```python
from build123d import *

# Parameters (mm, degrees)
SKETCH2_R      = 0.2
EXTRUDE1_DEPTH = 3
REVOLVE2_ANGLE = 45


with BuildPart() as part:
    # Sketch1 → Revolve1 (revolve)
    with BuildSketch(Plane.XY, mode=Mode.PRIVATE) as revolve1_sk:
        with BuildLine():
            Line((0, 0.3), (0, 10.7))
            Line((0, 10.7), (1, 10.7))
            Line((1, 10.7), (1, 11))
            Line((1, 11), (1.5, 11))
            ThreePointArc((1.5, 11), (1.853553391, 10.853553391), (2, 10.5))
            Line((2, 10.5), (2, 3.09445053))
            ThreePointArc((2, 3.09445053), (1.967707173, 2.917673834), (1.875, 2.763731616))
            ThreePointArc((1.875, 2.763731616), (1.75, 2.433012702), (1.875, 2.102293788))
            ThreePointArc((1.875, 2.102293788), (1.967707173, 1.948351569), (2, 1.771574874))
            Line((2, 1.771574874), (2, 0.5))
            ThreePointArc((2, 0.5), (1.853553391, 0.146446609), (1.5, 0))
            Line((1.5, 0), (1, 0))
            Line((1, 0), (1, 0.3))
            Line((1, 0.3), (0, 0.3))
        make_face()
    revolve(revolve1_sk.sketch.rotate(Axis((0, 0, 0), (0, -1, 0)), 270), axis=Axis((0, 0, 0), (0, -1, 0)))

    # Sketch2 → Extrude1 (add)
    with BuildSketch(Plane.XZ.offset(-0.3)):
        with Locations(Location((-0.75, 0, 0), (0, 0, 270))):
            Circle(SKETCH2_R)
        with Locations(Location((0.75, 0, 0), (0, 0, 90))):
            Circle(SKETCH2_R)
    extrude(amount=EXTRUDE1_DEPTH)

    # Sketch3 → Revolve2 (revolve, symmetric)
    with BuildSketch(Plane.XY) as revolve2_sk:
        with BuildLine():
            Line((0.99, 11.01), (0.99, -0.01))
            Line((0.99, -0.01), (1.5, -0.01))
            ThreePointArc((1.5, -0.01), (1.860624458, 0.139375542), (2.01, 0.5))
            Line((2.01, 0.5), (2.01, 1.771574874))
            ThreePointArc((2.01, 1.771574874), (1.977061317, 1.951887103), (1.8825, 2.108908166))
            ThreePointArc((1.8825, 2.108908166), (1.76, 2.433012702), (1.8825, 2.757117237))
            ThreePointArc((1.8825, 2.757117237), (1.977061317, 2.9141383), (2.01, 3.09445053))
            Line((2.01, 3.09445053), (2.01, 10.5))
            ThreePointArc((2.01, 10.5), (1.860624458, 10.860624458), (1.5, 11.01))
            Line((1.5, 11.01), (0.99, 11.01))
        make_face()
    revolve(axis=Axis((-0.01, 10.71, 0), (0, -1, 0)), revolution_arc=REVOLVE2_ANGLE / 2)
    revolve(revolve2_sk.sketch, axis=Axis((-0.01, 10.71, 0), (0, 1, 0)), revolution_arc=REVOLVE2_ANGLE / 2)


solid = part.part
```
Check sheet for the modelled part. Datum: model origin and axes. Units: mm. A direction names the side the tool comes from. Round coordinates to 2 decimals unless told otherwise and drop trailing zeros. Loops run counter-clockwise (first coordinate to the right, second up) from the corner with the lowest first, then second, coordinate; pieces in that order, holes last. Notation, with made-up numbers: (20.5, -32) - (46.5, -32) arc R31 ccw to (46.5, 6) - close; hole circle Ø9 at (75.5, 51). An arc over 180 degrees is marked (long way). Answer as a JSON object with one key per item and string values. Group by question number.
Q1. Scan lines: line 1 along Y through (x, z) = (-1.1, 0.55); line 2 along Z through (x, y) = (0, 10.8); line 3 along Z through (x, y) = (0, 10.9). Record each from-to range of solid material in increasing order. Write a range as [from, to].
Q2. Gauge pin test, flat ends, axial feed: P1, Ø2, axis at y = 0, z = 1.5, coming from the -X side; P2, Ø1.5, axis at x = -1, z = 1.5, coming from the +Y side; P3, Ø1.8, axis at x = 0, z = 0, coming from the +Y side. Record the tip position at first contact, or that the pin passes through.
Q3. Mould release check, pull along Z, two halves, no side actions. Record for faces 4 (the face through (-1, 11, 0.6)), 5 (the face through (0, 0.3, 0)), 6 (the face through (-2, 1, 0)): released by +Z, released by -Z, zero draft, split by the parting line, or undercut.
Q4. Sectioned sample at B-B, the plane x = 0. Enter the section's corners in (y, z) (3 decimals), plus the area to 3 significant figures.
Q5. Set-up check for faces 1 (the face through (-1, 0, -0.6)), 2 (the face through (-1, 10.85, 0.04)), 3 (the face through (-2, 7, 0)): record each of +Z, -Z, +X, -X, +Y, -Y from which the full face is reachable in a straight line by a thin tool's end or side.
Solution:
{
 "1": {"line 1": "y = [0, 11]", "line 2": "z = [-1.9, -1], [1, 1.9]", "line 3": "z = [-1.8, -1], [1, 1.8]"},
 "2": {"P1": "stops at x = -1.9", "P2": "stops at y = 11", "P3": "stops at y = 10.7"},
 "3": {"face 4": "zero draft", "face 5": "undercut", "face 6": "split by the parting line"},
 "4": {"outline": "(0, -1.5) arc R0.5 ccw to (0.5, -2) - (1.772, -2) arc R0.5 ccw to (2.102, -1.875) arc R0.5 cw to (2.764, -1.875) arc R0.5 ccw to (3.094, -2) - (10.5, -2) arc R0.5 ccw to (11, -1.5) - (11, -1) - (10.7, -1) - (10.7, 1) - (11, 1) - (11, 1.5) arc R0.5 ccw to (10.5, 2) - (3.094, 2) arc R0.5 ccw to (2.764, 1.875) arc R0.5 cw to (2.102, 1.875) arc R0.5 ccw to (1.772, 2) - (0.5, 2) arc R0.5 ccw to (0, 1.5) - (0, 1) - (0.3, 1) - (0.3, -1) - (0, -1) - close", "area": "42.3 mm²"},
 "5": {"face 1": "-X, -Y", "face 2": "+Y", "face 3": "+Y, -Y"}
}
